Source: three-view drawing plus pictorial views. Frame: mm from the lowest corner of the part. A direction names the side the tool comes from. Give positions to 0.01 mm unless a question says otherwise; leave off trailing zeros. Order: outer loops, then holes, each group sorted by start corner. A loop starts at its lowest first (then second) coordinate and runs counter-clockwise, first axis right, second up.
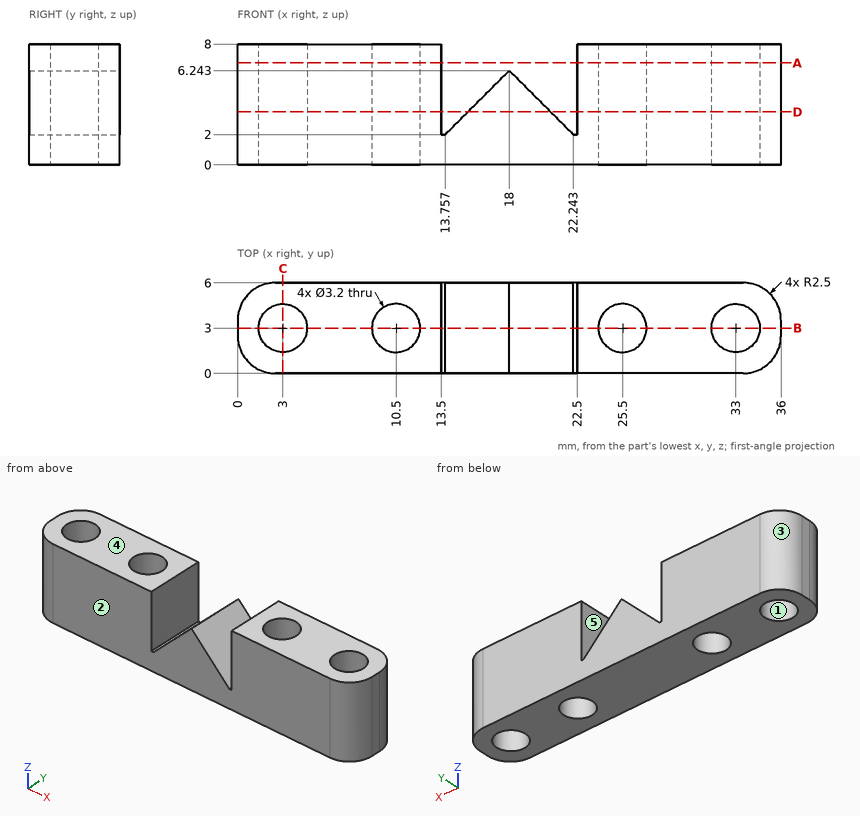
1) Section query A-A on z = 6.75. Output: boundary loops of the cut face in (x, y).
Checks:
outline: (0, 2.5) arc R2.5 ccw to (2.5, 0) - (13.5, 0) - (13.5, 6) - (2.5, 6) arc R2.5 ccw to (0, 3.5) - close; (22.5, 0) - (33.5, 0) arc R2.5 ccw to (36, 2.5) - (36, 3.5) arc R2.5 ccw to (33.5, 6) - (22.5, 6) - close; hole circle Ø3.2 at (3, 3); hole circle Ø3.2 at (10.5, 3); hole circle Ø3.2 at (25.5, 3); hole circle Ø3.2 at (33, 3)
2) Pull-direction query (X, two-part tool) for the marked faces 1, 2 and 3; classes: +X half, -X half, draft (parallel to the pull), parting line (faces both ways), or undercut.
Checks:
face 1: undercut
face 2: draft
face 3: -X half
3) Section query D-D on z = 3.5. Output: boundary loops of the cut face in (x, y), and give its area (3 significant figures).
Checks:
outline: (0, 2.5) arc R2.5 ccw to (2.5, 0) - (13.5, 0) - (13.5, 6) - (2.5, 6) arc R2.5 ccw to (0, 3.5) - close; (15.26, 0) - (20.74, 0) - (20.74, 6) - (15.26, 6) - close; (22.5, 0) - (33.5, 0) arc R2.5 ccw to (36, 2.5) - (36, 3.5) arc R2.5 ccw to (33.5, 6) - (22.5, 6) - close; hole circle Ø3.2 at (3, 3); hole circle Ø3.2 at (10.5, 3); hole circle Ø3.2 at (25.5, 3); hole circle Ø3.2 at (33, 3)
area: 157 mm2
4) First-contact query: pin 1 Ø3 at (y, z) = (0.5, 3) entering from -X. Flat tip, straight axial feed; report the tip coordinate or a pass-through.
Checks:
pin 1: stops at x = 0.05
5) Section query B-B on y = 3. Output: boundary loops of the cut face in (x, z).
Checks:
outline: (0, 0) - (1.4, 0) - (1.4, 8) - (0, 8) - close; (4.6, 0) - (8.9, 0) - (8.9, 8) - (4.6, 8) - close; (12.1, 0) - (23.9, 0) - (23.9, 8) - (22.5, 8) - (22.5, 2) - (22.24, 2) - (18, 6.24) - (13.76, 2) - (13.5, 2) - (13.5, 8) - (12.1, 8) - close; (27.1, 0) - (31.4, 0) - (31.4, 8) - (27.1, 8) - close; (34.6, 0) - (36, 0) - (36, 8) - (34.6, 8) - close
6) Section query C-C on x = 3. Output: boundary loops of the cut face in (y, z).
Checks:
outline: (0, 0) - (1.4, 0) - (1.4, 8) - (0, 8) - close; (4.6, 0) - (6, 0) - (6, 8) - (4.6, 8) - close
7) Reachability of the marked faces 4 and 5 from +Z, -Z, +X, -X, +Y, -Y: full face, straight path, thin tool, end or side. Return the list, or none.
Checks:
face 4: +Z, +X, -X, +Y, -Y
face 5: +Z, +Y, -Y
8) Ray query, L1, parallel to Y at x = 3, z = 4; L2, parallel to X at y = 5, z = 2.5; L3, parallel to Y at x = 25, z = 2. Return the intervals inside material, ascending.
Checks:
L1: y = 0 to 1.4, 4.6 to 6
L2: x = 0.5 to 13.5, 14.26 to 21.74, 22.5 to 35.5
L3: y = 0 to 1.48, 4.52 to 6
